Autodesk Inventor part; units mm, degrees
ref_plane "YZ Plane" through (0, 0, 0) normal (1, 0, 0) x (0, 1, 0)
ref_plane "XZ Plane" through (0, 0, 0) normal (0, 1, 0) x (-1, 0, 0)
ref_plane "XY Plane" through (0, 0, 0) normal (0, 0, 1) x (1, 0, 0)
sketch "Sketch1" plane through (0, 0, 0) normal (0, 0, 1) x (1, 0, 0)
  circle A0 centre (84.6636, 36.1746) radius 1.1933
  circle A1 centre (104.4626, 36.1746) radius 1.1933
  circle A2 centre (104.4626, 16.3756) radius 1.1933
  circle A3 centre (84.6636, 16.3756) radius 1.1933
  circle A4 centre (94.5631, 26.2751) radius 10
  circle A5 centre (94.5631, 26.2751) radius 14
  arc A6 (106.175, 34.0958) -> (102.3838, 37.887) centre (104.4626, 36.1746) ccw
  arc A7 (86.7424, 37.887) -> (82.9512, 34.0958) centre (84.6636, 36.1746) ccw
  arc A8 (82.9512, 18.4544) -> (86.7424, 14.6632) centre (84.6636, 16.3756) ccw
  arc A9 (102.3838, 14.6632) -> (106.175, 18.4544) centre (104.4626, 16.3756) ccw
  line L0 (80.5631, 26.2751) -> (108.5631, 26.2751) construction
  line L1 (104.5631, 26.2751) -> (100.935, 18.568)
  line L2 (104.5631, 26.2751) -> (100.935, 33.9822)
  circle A10 centre (94.0631, 26.2751) radius 9.5 construction
  point P0 (0, 0)
  dimension "d0" = 4
  dimension "d1" = 1.5
  dimension "d2" = 1.5
  dimension "d3" = 1.5
  dimension "d4" = 1.5
  dimension "d7" = 19
extrude "Extrusion1" add sketch "Sketch1" along normal blind 9 contours A0 A5 | A0 A5 A1 A2 A3 | A5 A0 | A0 A5 A7 | A6 A5 A1 | A5 A3 A8 | A5 A1 | A1 A5 | A5 A3 | A3 A5 | A5 A2 A9 | A5 A2 | A2 A5 | L2 A4 | A4 L1
hole "Hole1" at (104.4626, 16.3756, 0) at (84.6636, 16.3756, 0) at (84.6636, 36.1746, 0) at (104.4626, 36.1746, 0) direction (0, 0, 1) diameter 3.5 end through all
sketch "Sketch2" plane through (0, 0, 0) normal (1, 0, 0) x (0, 1, 0)
  line L0 (34.0958, 0) -> (18.4544, 0)
  line L1 (18.4544, 0) -> (18.4544, 9)
  line L2 (34.0958, 9) -> (18.4544, 9)
  line L3 (34.0958, 0) -> (34.0958, 9)
  line L4 (26.2751, 0) -> (26.2751, 9)
  point P0 (0, 0)
  point P1 (26.2751, 4.5)
hole "Hole2" at (0, 26.2751, 4.5) direction (1, 0, 0) diameter 4.6 depth 87.5 tip angle 118
properties part number "marker_holder"
Verification items for the finished model (mm, model axes). A direction names the side the tool comes from. Coordinates: 2 decimals unless noted, no trailing zeros. Loops run counter-clockwise (first coordinate to the right, second up) from the corner with the lowest first, then second, coordinate; pieces in that order, holes last. Notation, with made-up numbers: (-20, -28) -> (-8, -28) arc R32 cw to (-8, 6) -> close; hole circle Ø7 at (-3.75, 44). An arc over 180 degrees is marked (long way). Answer as a JSON object with one key per item and string values. Group by question number.
Item 1: Sectioned sample at D-D on y = 17.5. Record the boundary of the cut face in (x, z).
Item 2: Sectioned sample at C-C on y = 28. Record the boundary of the cut face in (x, z), plus the area to 3 significant figures.
Item 3: Sectioned sample at A-A on x = 89.25. Record the boundary of the cut face in (y, z).
Item 4: Scan lines: probe 1 along Y at (x, z) = (94.5, 2); probe 2 along Y at (x, z) = (105, 1.25); probe 3 along X at (y, z) = (32.5, 3.5). Record each from-to range of solid material in increasing order.
Item 5: Depth check by flat-ended pin: pin 1 (2 mm diameter, centred on x = 84.66, y = 36.17, fed in from +Z); pin 2 (4.5 mm diameter, centred on x = 104.46, y = 36.17, fed in from -Z); pin 3 (5 mm diameter, centred on x = 86, z = 5.5, fed in from +Y); pin 4 (1 mm diameter, centred on x = 99, z = 7.5, fed in from -Y). Enter the tip coordinate at first touch or a pass-through.
Item 6: Mould release check, pull along Y, two halves, no side actions. Record for faces 4 (the cylindrical face through (94.679, 12.276, 4.437)), 5 (the flat face through (104, 23, 9)), 6 (the cylindrical face through (85.728, 34.786, 4.563)): +Y half, -Y half, draft (parallel to the pull), parting line (faces both ways), or undercut.
Item 7: Tool access check on faces 1 (the cylindrical face through (82.7, 26.2, 2.2)), 2 (the cylindrical face through (108.563, 26.391, 4.437)), 3 (the flat face through (102.774, 30.075, 4.437)). Record the directions out of +Z, -Z, +X, -X, +Y, -Y that give a thin tool (end or side, any length) a straight path to the whole face; none if there is none.
Item 8: Sectioned sample at B-B on z = 4.5. Record the boundary of the cut face in (x, y) (3 decimals), plus the area to 3 significant figures.
Evaluation:
{
 "1": {"outline": "(82.22, 0) -> (83.32, 0) -> (83.32, 9) -> (82.22, 9) -> close; (86, 0) -> (89.77, 0) -> (89.77, 9) -> (86, 9) -> close; (99.36, 0) -> (103.12, 0) -> (103.12, 9) -> (99.36, 9) -> close; (105.8, 0) -> (106.91, 0) -> (106.91, 9) -> (105.8, 9) -> close"},
 "2": {"outline": "(80.67, 0) -> (84.71, 0) -> (84.71, 2.98) -> (80.67, 2.98) -> close; (80.67, 6.02) -> (84.71, 6.02) -> (84.71, 9) -> (80.67, 9) -> close; (103.75, 0) -> (108.46, 0) -> (108.46, 9) -> (103.75, 9) -> close", "area": "66.4 mm²"},
 "3": {"outline": "(13.32, 0) -> (17.8, 0) -> (17.8, 9) -> (13.32, 9) -> close; (34.75, 0) -> (39.23, 0) -> (39.23, 9) -> (34.75, 9) -> close"},
 "4": {"probe 1": "y = 12.28 to 16.28, 36.27 to 40.27", "probe 2": "y = 13.74 to 14.71, 18.04 to 34.51, 37.84 to 38.81", "probe 3": "x = 82.02 to 86.74, 101.63 to 107.1"},
 "5": {"pin 1": "passes through", "pin 2": "stops at z = 0", "pin 3": "stops at y = 38.89", "pin 4": "stops at y = 12.84"},
 "6": {"face 4": "-Y half", "face 5": "draft", "face 6": "undercut"},
 "7": {"face 1": "-X", "face 2": "+Z, -Z, +X", "face 3": "+Z, -Z"},
 "8": {"outline": "(80.753, 23.975) arc R14 ccw to (82.951, 18.454) arc R2.693 ccw (long way) to (86.742, 14.663) arc R14 ccw to (102.384, 14.663) arc R2.693 ccw (long way) to (106.175, 18.454) arc R14 ccw to (106.175, 34.096) arc R2.693 ccw (long way) to (102.384, 37.887) arc R14 ccw to (86.742, 37.887) arc R2.693 ccw (long way) to (82.951, 34.096) arc R14 ccw to (80.753, 28.575) -> (84.831, 28.575) arc R10 cw to (100.935, 33.982) -> (104.563, 26.275) -> (100.935, 18.568) arc R10 cw to (84.831, 23.975) -> close; hole circle Ø3.5 at (84.664, 16.376); hole circle Ø3.5 at (84.664, 36.175); hole circle Ø3.5 at (104.463, 16.376); hole circle Ø3.5 at (104.463, 36.175)", "area": "303 mm²"}
}
